Here's how the part is built. I have some questions about the finished solid (model axes, mm). Face numbers are marked on the shaded views. A direction names the side the tool comes from. Round coordinates to 2 decimals unless told otherwise and drop trailing zeros. Write each loop counter-clockwise with the first axis right and the second up, starting at its lowest first coordinate (ties: lowest second). Pieces come first, ordered by that corner, then holes. Notation, with made-up numbers: (5.5, 61) -> (53.5, 61) arc R22 ccw to (53.5, 80) -> close; hole circle Ø4 at (66, 56). An arc over 180 degrees is marked (long way). Answer as CSV lines item,"result".
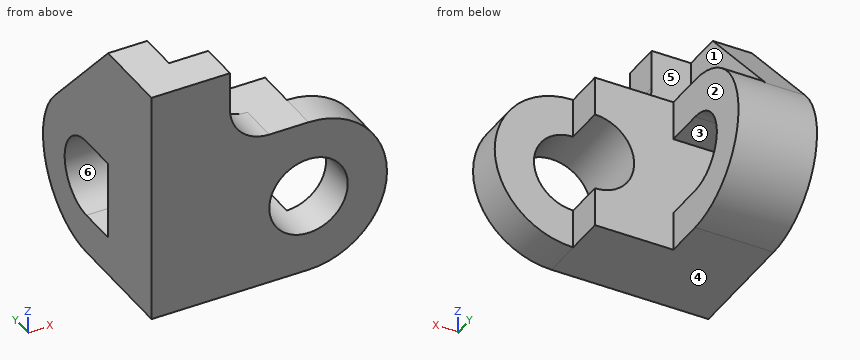
from build123d import *

# Parameters (mm, degrees)
SKETCH1_W           = 4
SKETCH1_H           = 2
BOSS_EXTRUDE1_DEPTH = 4
BOSS_EXTRUDE2_DEPTH = 1
SKETCH3_R           = 1
CUT_EXTRUDE1_DEPTH  = 3
SKETCH4_W           = 2
SKETCH4_H           = 1
BOSS_EXTRUDE3_DEPTH = 2
SKETCH5_W           = 1
SKETCH5_H           = 2
BOSS_EXTRUDE4_DEPTH = 1
BOSS_EXTRUDE5_DEPTH = 1
BOSS_EXTRUDE6_DEPTH = 1


with BuildPart() as part:
    # Sketch1 → Boss-Extrude1 (new body)
    with BuildSketch(Plane.XY):
        Rectangle(SKETCH1_W, SKETCH1_H)
    extrude(amount=BOSS_EXTRUDE1_DEPTH)

    # Sketch2 → Boss-Extrude2 (add)
    with BuildSketch(Plane.XZ.offset(1)):
        with BuildLine():
            Line((2, 4), (2, 0))
            ThreePointArc((2, 0), (4, 2), (2, 4))
        make_face()
    extrude(amount=-BOSS_EXTRUDE2_DEPTH)

    # Sketch3 → Cut-Extrude1 (cut, through all)
    with BuildSketch(Plane(origin=(0, 1, 0), x_dir=(1, 0, 0), z_dir=(0, 1, 0))):
        with Locations((2, -2)):
            Circle(SKETCH3_R)
    extrude(amount=-CUT_EXTRUDE1_DEPTH, mode=Mode.SUBTRACT)

    # Sketch4 → Boss-Extrude3 (add)
    with BuildSketch(Plane.ZY.offset(2)):
        with Locations((5, -0.5)):
            Rectangle(SKETCH4_W, SKETCH4_H)
        with BuildLine():
            Line((0, 1), (0, 2))
            ThreePointArc((0, 2), (2, 4), (4, 2))
            Line((4, 2), (4, 1))
            Line((4, 1), (3, 1))
            Line((3, 1), (3, 2))
            ThreePointArc((3, 2), (2, 3), (1, 2))
            Line((1, 2), (1, 1))
            Line((1, 1), (0, 1))
        make_face()
    extrude(amount=-BOSS_EXTRUDE3_DEPTH)

    # Sketch5 → Boss-Extrude4 (add)
    with BuildSketch(Plane(origin=(0, 0, 0), x_dir=(1, 0, 0), z_dir=(0, 1, 0))):
        with Locations((-1.5, -5)):
            Rectangle(SKETCH5_W, SKETCH5_H)
    extrude(amount=BOSS_EXTRUDE4_DEPTH)

    # Sketch6 → Boss-Extrude5 (add)
    with BuildSketch(Plane.ZY.offset(2)):
        with BuildLine():
            Line((3.365358974, 3.461435894), (6, 1))
            Line((6, 1), (4, 1))
            Line((4, 1), (4, 2))
            ThreePointArc((4, 2), (3.834491475, 2.796643601), (3.365358974, 3.461435894))
        make_face()
    extrude(amount=-BOSS_EXTRUDE5_DEPTH)

    # Sketch7 → Boss-Extrude6 (add)
    with BuildSketch(Plane(origin=(0, 0, 0), x_dir=(1, 0, 0), z_dir=(0, 1, 0))):
        with BuildLine():
            Line((1, -4), (0, -4))
            Line((0, -4), (0, -5))
            ThreePointArc((0, -5), (0.292893219, -4.292893219), (1, -4))
        make_face()
    extrude(amount=-BOSS_EXTRUDE6_DEPTH)


solid = part.part
Item 1: Suppose I cut it at D-D, the plane y = 2.7. List the corners of the cut face in (x, z) for me, then the cut area to 3 significant figures.
Results found:
outline,"(-2, 0.13) -> (0, 0.13) -> (0, 1.29) -> (-2, 1.29) -> close; (-2, 2.71) -> (0, 2.71) -> (0, 3.87) -> (-1, 3.87) -> (-1, 4.18) -> (-2, 4.18) -> close"
area,"4.94 mm²"
Item 2: I need wall thicknesses on L1, parallel to X at y = -0.1, z = 2; L2, parallel to Z at x = 2, y = -0.4; L3, parallel to Y at x = -0.35, z = 1.95. Which ranges of each line are inside material? Lowest first, please.
Results found:
L1,"x = -2 to 1, 3 to 4"
L2,"z = 0 to 1, 3 to 4"
L3,"y = -1 to 1, 3 to 4"
Item 3: Suppose I cut it at C-C, the plane x = -0.15. List the corners of the cut face in (y, z) for me, then the cut area to 3 significant figures.
Results found:
outline,"(-1, 0) -> (2, 0) arc R2 ccw to (2, 4) -> (0, 4) -> (0, 6) -> (-1, 6) -> close; hole (1, 1) -> (2, 1) arc R1 ccw to (2, 3) -> (1, 3) -> close"
area,"16.7 mm²"
Item 4: For the marked faces 1, 2 and 3, which set-ups out of +Z, -Z, +X, -X, +Y, -Y let a thin tool reach every point of the face, with its end or its side?
Results found:
face 1,"+Z, +X, +Y"
face 2,"+Z, -Z, +X, +Y"
face 3,"+X, -X"
Item 5: If we mould it in two halves opening along Y, with no side actions, what happens to the marked faces 4, 5 and 6? For each: pulls with the +Y half, pulls with the -Y half, needs draft (parallel to the pull), parting line crosses it, or undercut.
Results found:
face 4,"needs draft"
face 5,"pulls with the +Y half"
face 6,"undercut"
Item 6: Suppose I cut it at A-A, the plane z = 2. List the corners of the cut face in (x, y) for me, then the cut area to 3 significant figures.
Results found:
outline,"(-2, -1) -> (1, -1) -> (1, 1) -> (-2, 1) -> close; (-2, 3) -> (0, 3) -> (0, 4) -> (-2, 4) -> close; (3, -1) -> (4, -1) -> (4, 0) -> (3, 0) -> close"
area,"9.00 mm²"
Item 7: Will these pins go through, and if not, where does the flat tip stop? pin 1 (1.6 mm diameter, centred on x = 2, z = 2, fed in from +Y); pin 2 (3 mm diameter, centred on y = 2, z = 4, fed in from +X); pin 3 (2 mm diameter, centred on x = 2.5, z = 2, fed in from +Y); pin 4 (0.5 mm diameter, centred on x = -1, y = 1.5, fed in from +Z).
Results found:
pin 1,"passes through"
pin 2,"stops at x = 2"
pin 3,"stops at y = 0"
pin 4,"stops at z = 5.73"
Item 8: Suppose I cut it at B-B, the plane y = 0.3. List the corners of the cut face in (x, z) for me, then the cut area to 3 significant figures.
Results found:
outline,"(-2, 0) -> (2, 0) -> (2, 1) arc R1 cw to (2, 3) -> (2, 4) -> (-1, 4) -> (-1, 6) -> (-2, 6) -> close"
area,"16.4 mm²"
